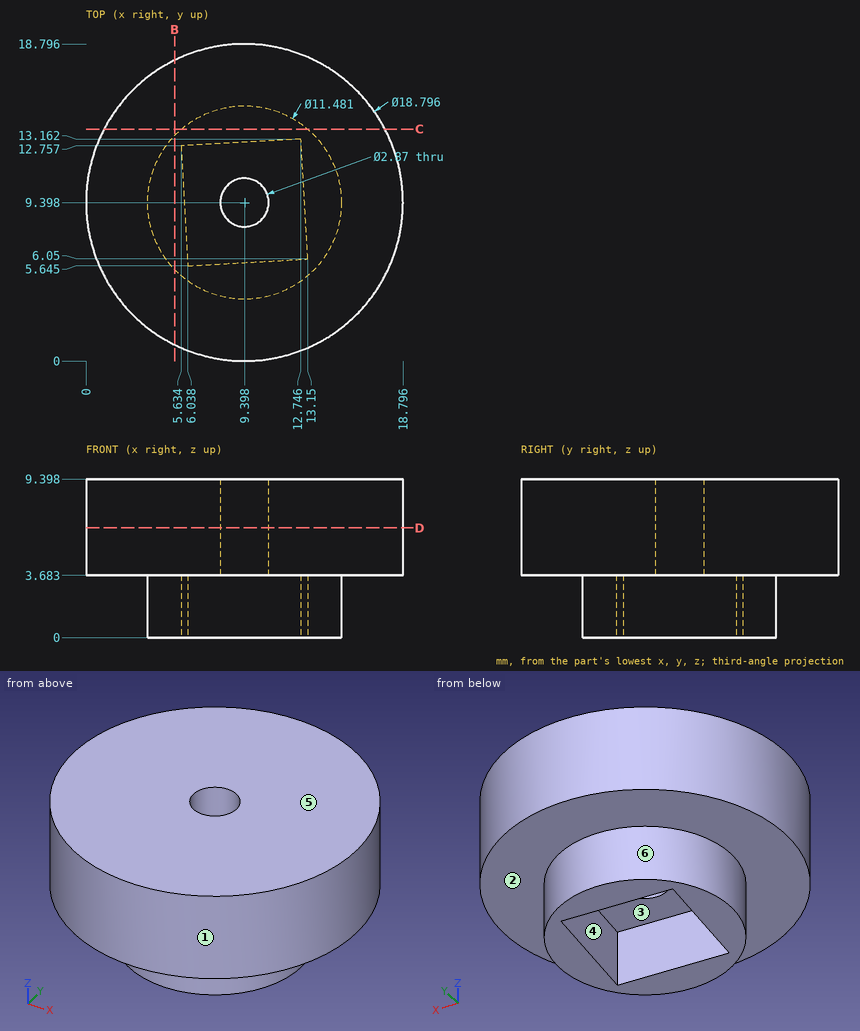
Answer from the drawing. Dimensions are ordinates in mm from the lowest x, y and z of the part. A direction names the side the tool comes from. Give positions to 0.01 mm unless a question says otherwise; leave off trailing zeros. Loops run counter-clockwise (first coordinate to the right, second up) from the corner with the lowest first, then second, coordinate; pieces in that order, holes last.
Item 1: The part is cut by section C-C (y = 13.75). Write down the section's boundary in (x, z) (1 decimal), and give its area (3 significant figures).
Item 2: The part is cut by section B-B (x = 5.25). Write down the section's boundary in (y, z) (1 decimal).
Item 3: Find the intervals of material crossed by line 1 along Z through (x, y) = (14.5, 13.25); line 2 along X through (y, z) = (10, 9.25) (1 decimal); line 3 along Y through (x, z) = (11.75, 2) (1 decimal), in increasing order.
Item 4: The part is cut by section D-D (z = 6.5). Write down the section's boundary in (x, y) (1 decimal), and give its area (3 significant figures).
Item 5: For the marked faces 5 and 6, determine the directions among +Z, -Z, +X, -X, +Y, -Y from which every point of the face is accessible in a straight line to the end or side of a thin tool.
Item 6: Each of these flat-tipped pins is pushed along its axis until it touches: pin 1 Ø2 at (x, z) = (13, 3.5) entering from -Y; pin 2 Ø3 at (x, z) = (15, 7.5) entering from +Y; pin 3 Ø2.5 at (x, y) = (11, 9) entering from -Z. Where does it stop, or does it pass through?
Item 7: The mould has two halves that part along Y. Classify the marked faces 1, 2, 3 and 4: released by +Y, released by -Y, zero draft, split by the parting line, or undercut.
Taken from the geometry:
1. outline: (1.1, 3.7) - (5.7, 3.7) - (5.7, 0) - (13.1, 0) - (13.1, 3.7) - (17.7, 3.7) - (17.7, 9.4) - (1.1, 9.4) - close
1. area: 123 mm2
2. outline: (1, 3.7) - (5.4, 3.7) - (5.4, 0) - (13.4, 0) - (13.4, 3.7) - (17.8, 3.7) - (17.8, 9.4) - (1, 9.4) - close
3. line 1: z = 3.68 to 9.4
3. line 2: x = 0 to 8.1, 10.7 to 18.8
3. line 3: y = 4.2 to 6, 13.1 to 14.6
4. outline: circle Ø18.8 at (9.4, 9.4); hole circle Ø2.9 at (9.4, 9.4)
4. area: 271 mm2
5. face 5: +Z, +X, -X, +Y, -Y
5. face 6: -Z
6. pin 1: stops at y = 0.37
6. pin 2: stops at y = 17.85
6. pin 3: stops at z = 3.68
7. face 1: split by the parting line
7. face 2: zero draft
7. face 3: undercut
7. face 4: undercut
